```python
from build123d import *

# Parameters (mm, degrees)
SKETCH1_W               = 120
SKETCH1_H               = 32
EXTRUDE1_DEPTH          = 75
CUT_EXTRUDE4_START      = 8
SKETCH2_OUTSIDE_W       = 151.016
SKETCH2_OUTSIDE_H       = 63.016
CUT_EXTRUDE4_DEPTH      = 68
EXTRUDE7_DEPTH          = 36.5252
SKETCH6_R               = 6.35
SKETCH6_R_2             = 4.1021
EXTRUDE4_DEPTH          = 33
SKETCH8_OUTSIDE_W       = 151.016
SKETCH8_OUTSIDE_H       = 106.016
EXTRUDE8_DEPTH          = 33
SKETCH9_R               = 4.1021
CUT_EXTRUDE1_DEPTH      = 43.0000001
FILLET6_R               = 2
CUT_EXTRUDE2_DEPTH      = 17
CUT_EXTRUDE2_DEPTH_BACK = 17.0000001
SKETCH16_OUTSIDE_W      = 136.204
SKETCH16_OUTSIDE_H      = 58.204
CUT_EXTRUDE7_DEPTH      = 43.0000001


with BuildPart() as part:
    # Sketch1 → Extrude1 (new body)
    with BuildSketch(Plane.XY.offset(3)):
        with Locations((60, 0)):
            Rectangle(SKETCH1_W, SKETCH1_H)
    extrude(amount=EXTRUDE1_DEPTH)

    # Sketch2 outside → Cut-Extrude4 (cut, through all)
    with BuildSketch(Plane.XY.offset(3).offset(CUT_EXTRUDE4_START)):
        with Locations((60, 0)):
            Rectangle(SKETCH2_OUTSIDE_W, SKETCH2_OUTSIDE_H)
        with BuildLine():
            Line((0, 16), (82.254775894, 16))
            Line((82.254775894, 16), (91.071137947, 7.183637947))
            ThreePointArc((91.071137947, 7.183637947), (92.873715179, 5.979194347), (95, 5.55625))
            Line((95, 5.55625), (120, 5.55625))
            Line((120, 5.55625), (120, 0.55625))
            Line((120, 0.55625), (95, 0.55625))
            ThreePointArc((95, 0.55625), (89.44375, -5), (95, -10.55625))
            Line((95, -10.55625), (120, -10.55625))
            Line((120, -10.55625), (120, -16))
            Line((120, -16), (0, -16))
            Line((0, -16), (0, -11.1125))
            Line((0, -11.1125), (75, -11.1125))
            ThreePointArc((75, -11.1125), (86.1125, 0), (75, 11.1125))
            Line((75, 11.1125), (0, 11.1125))
            Line((0, 11.1125), (0, 16))
        make_face(mode=Mode.SUBTRACT)
    extrude(amount=CUT_EXTRUDE4_DEPTH, mode=Mode.SUBTRACT)

    # Sketch7 → Extrude7 (cut)
    with BuildSketch(Plane.XY):
        with BuildLine():
            Line((95, 5.55625), (120, 5.55625))
            Line((120, 5.55625), (133.084512724, 5.55625))
            Line((133.084512724, 5.55625), (133.084512724, 22.23007271))
            Line((133.084512724, 22.23007271), (82.254775894, 22.23007271))
            Line((82.254775894, 22.23007271), (82.254775894, 16))
            Line((82.254775894, 16), (91.071137947, 7.183637947))
            ThreePointArc((91.071137947, 7.183637947), (92.873715179, 5.979194347), (95, 5.55625))
        make_face()
    extrude(amount=EXTRUDE7_DEPTH, mode=Mode.SUBTRACT)

    # Sketch6 → Extrude4 (cut, through all)
    with BuildSketch(Plane(origin=(0, 16, 0), x_dir=(1, 0, 0), z_dir=(0, 1, 0))):
        with Locations((26.4, -30.9)):
            Circle(SKETCH6_R)
        with Locations((102.4, -30.9)):
            Circle(SKETCH6_R_2)
    extrude(amount=-EXTRUDE4_DEPTH, mode=Mode.SUBTRACT)

    # Sketch8 outside → Extrude8 (cut, through all)
    with BuildSketch(Plane(origin=(0, 16, 0), x_dir=(1, 0, 0), z_dir=(0, 1, 0))):
        with Locations((60, -40.5)):
            Rectangle(SKETCH8_OUTSIDE_W, SKETCH8_OUTSIDE_H)
        with BuildLine():
            Line((17.594193491, -41.157475527), (2.4, -10))
            Line((2.4, -10), (2.4, 17.886579673))
            Line((2.4, 17.886579673), (88.4, 17.886579673))
            Line((88.4, 17.886579673), (88.4, -12.2))
            ThreePointArc((88.4, -12.2), (90.259871939, -16.690128061), (94.75, -18.55))
            Line((94.75, -18.55), (102.875, -18.55))
            ThreePointArc((102.875, -18.55), (109.610192091, -21.339807909), (112.4, -28.075))
            Line((112.4, -28.075), (112.4, -32.475))
            ThreePointArc((112.4, -32.475), (109.610192091, -39.210192091), (102.875, -42))
            Line((102.875, -42), (18.942424158, -42))
            ThreePointArc((18.942424158, -42), (18.147506958, -41.772048209), (17.594193491, -41.157475527))
        make_face(mode=Mode.SUBTRACT)
    extrude(amount=-EXTRUDE8_DEPTH, mode=Mode.SUBTRACT)

    # Sketch9 → Cut-Extrude1 (cut, through all)
    with BuildSketch(Plane.XY):
        with Locations((13, 0)):
            Circle(SKETCH9_R)
        with Locations((75, 0)):
            Circle(SKETCH9_R)
    extrude(amount=CUT_EXTRUDE1_DEPTH, mode=Mode.SUBTRACT)

    # Fillet6
    fillet6_edges = [part.edges().sort_by_distance(p)[0] for p in [
        (38.943829021, 11.1125, 11),
        (86.1125, 0, 11),
        (38.943829021, -11.1125, 11),
    ]]
    fillet(fillet6_edges, radius=FILLET6_R)

    # Sketch10 → Cut-Extrude2 (cut, two sides)
    with BuildSketch(Plane(origin=(0, 0, 0), x_dir=(1, 0, 0), z_dir=(0, 1, 0))) as cut_extrude2_sk:
        with BuildLine():
            Line((32, -14.35), (56, -14.35))
            ThreePointArc((56, -14.35), (60.490128061, -12.490128061), (62.35, -8))
            Line((62.35, -8), (62.35, 20.451290564))
            Line((62.35, 20.451290564), (25.65, 20.451290564))
            Line((25.65, 20.451290564), (25.65, -8))
            ThreePointArc((25.65, -8), (27.509871939, -12.490128061), (32, -14.35))
        make_face()
    extrude(amount=CUT_EXTRUDE2_DEPTH, mode=Mode.SUBTRACT)
    extrude(cut_extrude2_sk.sketch, amount=-CUT_EXTRUDE2_DEPTH_BACK, mode=Mode.SUBTRACT)

    # Sketch16 outside → Cut-Extrude7 (cut, through all)
    with BuildSketch(Plane.XY):
        with Locations((57.4, 0)):
            Rectangle(SKETCH16_OUTSIDE_W, SKETCH16_OUTSIDE_H)
        with BuildLine():
            Line((2.4, 8.0625), (2.4, -8.0625))
            ThreePointArc((2.4, -8.0625), (4.724839924, -13.675160076), (10.3375, -16))
            Line((10.3375, -16), (122.688337856, -16))
            Line((122.688337856, -16), (122.688337856, 16))
            Line((122.688337856, 16), (10.3375, 16))
            ThreePointArc((10.3375, 16), (4.724839924, 13.675160076), (2.4, 8.0625))
        make_face(mode=Mode.SUBTRACT)
    extrude(amount=CUT_EXTRUDE7_DEPTH, mode=Mode.SUBTRACT)

    # Cut-Sweep1: sweep along a path in Sketch19
    with BuildLine(Plane.XZ.offset(16)) as cut_sweep1_path:
        ThreePointArc((88.4, 3), (90.498611985, 8.066497517), (95.565109502, 10.165109502))
    # Sketch17 → Cut-Sweep1 (sweep, cut)
    with BuildSketch(Plane(origin=(0, 0, 3), x_dir=(-1, 0, 0), z_dir=(0, 0, -1))):
        with BuildLine():
            Line((-80.4625, -16), (-80.4625, -23.337063984))
            Line((-80.4625, -23.337063984), (-92.369, -23.337063984))
            Line((-92.369, -23.337063984), (-92.369, -8.0625))
            Line((-92.369, -8.0625), (-88.4, -8.0625))
            ThreePointArc((-88.4, -8.0625), (-86.075160076, -13.675160076), (-80.4625, -16))
        make_face()
    sweep(path=cut_sweep1_path.line, mode=Mode.SUBTRACT)


solid = part.part
```
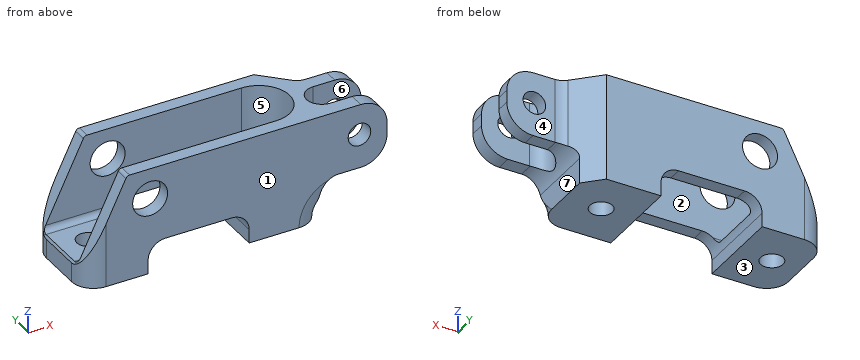
Build history of the part. All positions in model axes, mm. Face numbers are marked on the shaded views. A direction names the side the tool comes from. Give positions to 0.01 mm unless a question says otherwise; leave off trailing zeros. Loops run counter-clockwise (first coordinate to the right, second up) from the corner with the lowest first, then second, coordinate; pieces in that order, holes last. Notation, with made-up numbers: (65.5, -0.75) -> (85.5, -0.75) arc R36 ccw to (85.5, 37.25) -> close; hole circle Ø6 at (88.25, -39.5). An arc over 180 degrees is marked (long way). One line per question, with ' | ' between items.
Q1. Drill centre lines: line 1 along X through (y, z) = (0, 7.75); line 2 along Y through (x, z) = (101.5, 40.5); line 3 along Y through (x, z) = (13, 9). Where is each one in solid material? Low to high. Write a range as [from, to].
Filled sheet:
line 1: x = [2.4, 8.9], [17.1, 25.65], [62.35, 70.9], [79.1, 88.4] | line 2: y = [-16, -10.56], [0.56, 5.56] | line 3: y = [-16, -4.1], [4.1, 16]
Q2. Cut at C-C, the plane x = 93. Write the cut outline in (y, z).
Filled sheet:
outline: (-16, 18.3) -> (-10.18, 18.3) -> (-10.18, 42) -> (-16, 42) -> close; (0.18, 18.3) -> (5.93, 18.3) -> (5.93, 42) -> (0.18, 42) -> close
Q3. Cut at B-B, the plane z = 30.9. Count the separate pieces of the cut face and the enclosed holes in it, plus the area to 3 significant figures.
Filled sheet:
separate pieces: 5 | enclosed holes: 0 | area: 902 mm²
Q4. Cut at A-A, the plane x = 13. Write the cut outline in (y, z).
Filled sheet:
outline: (-16, 3) -> (-4.1, 3) -> (-4.1, 11) -> (-9.11, 11) arc R2 cw to (-11.11, 13) -> (-11.11, 31.74) -> (-16, 31.74) -> close; (4.1, 3) -> (16, 3) -> (16, 31.74) -> (11.11, 31.74) -> (11.11, 13) arc R2 cw to (9.11, 11) -> (4.1, 11) -> close
Q5. Drop flat-ended pins along their axis: pin 1 (4.5 mm diameter, centred on x = 97, y = -13.5, fed in from -Z); pin 2 (9.5 mm diameter, centred on x = 75, y = 0, fed in from +Z); pin 3 (13 mm diameter, centred on x = 102.4, z = 30.9, fed in from +Y); pin 4 (7.5 mm diameter, centred on x = 13, y = 0, fed in from -Z) (1 decimal). Give the stop position or say it passes through.
Filled sheet:
pin 1: stops at z = 18.55 | pin 2: stops at z = 11 | pin 3: stops at y = 5.56 | pin 4: passes through
Q6. Pull direction Y, two halves, no side cores. Call the marked faces 1, 2 and 3: pulls with the +Y half, pulls with the -Y half, needs draft (parallel to the pull), parting line crosses it, or undercut.
Filled sheet:
face 1: pulls with the -Y half | face 2: undercut | face 3: needs draft
Q7. Tool access for the marked faces 4, 5, 6 and 7: list every direction of +Z, -Z, +X, -X, +Y, -Y with a clear straight run to the whole face (end or side of a thin tool).
Filled sheet:
face 4: +Z, -Z, +X, +Y | face 5: +Z, -X | face 6: +Z, -Z, +X | face 7: -Z, +X, +Y, -Y
